```python
from build123d import *

# Parameters (mm, degrees)
PAD_DEPTH    = 9
SKETCH001_R  = 1.5
PAD001_DEPTH = 7
SKETCH002_R  = 2
POCKET_DEPTH = 2
SKETCH003_R  = 3
PAD002_DEPTH = 3
FILLET_R     = 2.75
CHAMFER_SIZE = 8


with BuildPart() as part:
    # Sketch → Pad (new body)
    with BuildSketch(Plane.XY):
        Polygon((6.5, -11), (6.5, 33), (5, 33), (5, 43), (-5, 43), (-5, 33), (-6.5, 33), (-6.5, -11), align=None)
    extrude(amount=PAD_DEPTH)

    # Sketch001 → Pad001 (join, symmetric)
    with BuildSketch(Plane.YZ):
        with Locations((40, 1.5)):
            Circle(SKETCH001_R)
    extrude(amount=PAD001_DEPTH, both=True)

    # Sketch002 (on Face4 of Pad001) → Pocket (cut)
    with BuildSketch(Plane(origin=(0, 0, 0), x_dir=(1, 0, 0), z_dir=(0, 0, -1))):
        with Locations((0, 1)):
            Circle(SKETCH002_R)
    extrude(amount=-POCKET_DEPTH, mode=Mode.SUBTRACT)

    # Sketch003 (on Face4 of Pocket) → Pad002 (join)
    with BuildSketch(Plane(origin=(0, 0, 0), x_dir=(1, 0, 0), z_dir=(0, 0, -1))):
        with Locations((0, -23)):
            Circle(SKETCH003_R)
    extrude(amount=PAD002_DEPTH)

    # Fillet
    fillet_edges = [part.edges().sort_by_distance(p)[0] for p in [
        (-3, 23, -3),
    ]]
    fillet(fillet_edges, radius=FILLET_R)

    # Chamfer
    chamfer_edges = [part.edges().sort_by_distance(p)[0] for p in [
        (0, -11, 9),
    ]]
    chamfer(chamfer_edges, length=CHAMFER_SIZE)


solid = part.part
```
The listing builds one solid part. Answer for the finished solid, in the listing's coordinates (mm). A direction names the side the tool comes from. Coordinates: 2 decimals unless noted, no trailing zeros. Write each loop counter-clockwise with the first axis right and the second up, starting at its lowest first coordinate (ties: lowest second). Pieces come first, ordered by that corner, then holes. Notation, with made-up numbers: (29, 79) - (69, 79) arc R10 ccw to (69, 98) - close; hole circle Ø6 at (34.25, 22). An arc over 180 degrees is marked (long way). Return JSON: item names as keys, results as strings. Group by question number.
1. A cutting plane is placed at B-B, the plane x = -6. Determine the outline of the cut face in (y, z).
2. A cutting plane is placed at D-D, the plane y = -1. Determine the outline of the cut face in (x, z), plus the area to 3 significant figures.
3. A cutting plane is placed at C-C, the plane z = 3.5. Determine the outline of the cut face in (x, y), plus the area to 4 significant figures.
4. A cutting plane is placed at A-A, the plane z = 1.5. Determine the outline of the cut face in (x, y).
5. Which of the six approach directions +Z, -Z, +X, -X, +Y, -Y give full straight-line access (tool end or side, diameter ignored) to faces 1 (the flat face through (0, -1, 2)), 2 (the flat face through (-6, 33, 4)), 3 (the flat face through (-6.5, 11, 4))?
6. Determine the mould class of faces 4 (the flat face through (-0.1, -11, 0.5)), 5 (the cylindrical face through (6.01, 38.5, 1.57)), 6 (the flat face through (0, 16, 0)) for opening direction Y: released by +Y, released by -Y, zero draft, split by the parting line, or undercut.
7. Straight lines are drawn through the part: L1, parallel to Y at x = 0, z = 0.5; L2, parallel to X at y = -1, z = 1.25; L3, parallel to X at y = 27, z = 0.75. For each, find the intervals that lie inside material, in ascending order.
8. Given pin 1 (0.8 mm diameter, centred on x = -6, z = 4.5, fed in from +Y); pin 2 (4.5 mm diameter, centred on y = 37, z = 6, fed in from +X); pin 3 (5 mm diameter, centred on y = -3.5, z = -1.5, fed in from +X), each flat-ended and moving along its own axis, determine where each tip first touches the part or whether it passes through.
Ans:
{
 "1": {"outline": "(-11, 0) - (33, 0) - (33, 9) - (-3, 9) - (-11, 1) - close; circle Ø3 at (40, 1.5)"},
 "2": {"outline": "(-6.5, 0) - (-2, 0) - (-2, 2) - (2, 2) - (2, 0) - (6.5, 0) - (6.5, 9) - (-6.5, 9) - close", "area": "109 mm²"},
 "3": {"outline": "(-6.5, -8.5) - (6.5, -8.5) - (6.5, 33) - (5, 33) - (5, 43) - (-5, 43) - (-5, 33) - (-6.5, 33) - close", "area": "639.5 mm²"},
 "4": {"outline": "(-7, 38.5) - (-5, 38.5) - (-5, 33) - (-6.5, 33) - (-6.5, -10.5) - (6.5, -10.5) - (6.5, 33) - (5, 33) - (5, 38.5) - (7, 38.5) - (7, 41.5) - (5, 41.5) - (5, 43) - (-5, 43) - (-5, 41.5) - (-7, 41.5) - close; hole circle Ø4 at (0, -1)"},
 "5": {"face 1": "-Z", "face 2": "+Z, -Z, -X", "face 3": "+Z, -Z, -X, -Y"},
 "6": {"face 4": "released by -Y", "face 5": "undercut", "face 6": "zero draft"},
 "7": {"L1": "-11 to -3, 1 to 43", "L2": "-6.5 to -2, 2 to 6.5", "L3": "-6.5 to 6.5"},
 "8": {"pin 1": "y = 33", "pin 2": "x = 5", "pin 3": "x = 6.5"}
}
